Design review of the part built by this model. Coordinates are the model's own, in mm. A direction names the side the tool comes from. Round coordinates to 2 decimals unless told otherwise and drop trailing zeros. Order: outer loops, then holes, each group sorted by start corner. A loop starts at its lowest first (then second) coordinate and runs counter-clockwise, first axis right, second up.
Autodesk Inventor part; units mm, degrees
ref_plane "YZ Plane" through (0, 0, 0) normal (1, 0, 0) x (0, 1, 0)
ref_plane "XZ Plane" through (0, 0, 0) normal (0, 1, 0) x (-1, 0, 0)
ref_plane "XY Plane" through (0, 0, 0) normal (0, 0, 1) x (1, 0, 0)
sketch "Sketch4" plane through (0, 0, 0) normal (1, 0, 0) x (0, 1, 0)
  line L0 (0, 0) -> (3, 0)
  line L1 (3, 0) -> (3, -4.5)
  line L2 (3, -4.5) -> (0, -4.5)
  line L3 (0, -4.5) -> (0, 0)
  dimension "d21" = 3
  dimension "d22" = 4.5
extrude "Extrusion2" add sketch "Sketch4" along normal blind 100
sketch "Sketch5" plane through (0, 3, 0) normal (0, 1, 0) x (1, 0, 0)
  circle A0 centre (2.25, 2.25) radius 1.5
  circle A1 centre (96.8723, 2.25) radius 1.5
  line L0 (0, 4.5) -> (0, 0) construction
  line L1 (0, 0) -> (100, 0) construction
  dimension "d25" = 3
  dimension "d26" = 3
  dimension "d27" = 2.25
  dimension "d28" = 2.25
  dimension "d29" = 4.5
hole "Hole2" at (2.25, 3, -2.25) at (96.8723, 3, -2.25) direction (0, -1, 0) diameter 3.4 depth 8.8 tip angle 118
sketch "Sketch6" plane through (0, 3, 0) normal (0, 1, 0) x (1, 0, 0)
  line L0 (7.5, 1.15) -> (92.5, 1.15)
  line L1 (92.5, 1.15) -> (92.5, 3.35)
  line L2 (92.5, 3.35) -> (7.5, 3.35)
  line L3 (7.5, 3.35) -> (7.5, 1.15)
  line L4 (0, 4.5) -> (100, 4.5)
  line L5 (0, 0) -> (100, 0)
  line L6 (0, 4.5) -> (0, 0)
  dimension "d37" = 85
  dimension "d38" = 2.2
  dimension "d39" = 4.5
  dimension "d40" = 1.15
  dimension "d41" = 7.5
extrude "Extrusion3" cut sketch "Sketch6" against normal blind 100
sketch "Sketch7" plane through (0, 0, 0) normal (0, 0, 1) x (1, 0, 0)
  line L0 (0, 0) -> (100, 0)
  line L1 (100, 0) -> (100, 3)
  line L2 (100, 3) -> (0, 3)
  line L3 (0, 3) -> (0, 0)
extrude "Extrusion4" add sketch "Sketch7" along normal blind 8
sketch "Sketch8" plane through (0, 3, -4.5) normal (0, 1, 0) x (1, 0, 0)
  line L0 (11, -9.5) -> (89, -9.5) construction
  line L1 (0, 0) -> (0, -12.5)
  line L2 (-1, -16) -> (89, -16) construction
  line L3 (-1, -17) -> (89, -17) construction
  line L4 (89, -15) -> (-1, -15) construction
  arc A0 (-1, -15) -> (-1, -17) centre (-1, -16) ccw construction
  arc A1 (89, -17) -> (89, -15) centre (89, -16) ccw construction
  circle A2 centre (11, -9.5) radius 1
  circle A3 centre (89, -9.5) radius 1
  circle A4 centre (82.5, -9.5) radius 1
  circle A5 centre (17.5, -9.5) radius 1
  point P0 (0, -4.5)
  point P1 (50, -9.5)
  point P2 (44, -16)
  dimension "d47" = 78
  dimension "d48" = 50
  dimension "d49" = 2
  dimension "d50" = 90
  dimension "d51" = 6.5
  dimension "d54" = 9.5
  dimension "d55" = 2
  dimension "d56" = 2
  dimension "d57" = 2
  dimension "d58" = 2
  dimension "d59" = 6.5
  dimension "d60" = 6.5
sketch "Sketch9" plane through (0, 0, -4.5) normal (0, -1, 0) x (1, 0, 0)
  point P0 (0, 4.5)
sketch "Sketch10" plane through (0, 0, -4.5) normal (0, -1, 0) x (1, 0, 0)
  point P0 (0, 4.5)
hole "Hole3" at (11, 3, 5) at (17.5, 3, 5) at (82.5, 3, 5) at (89, 3, 5) direction (0, -1, 0) diameter 1.221 depth 5.3 tip angle 118
chamfer "Chamfer1" distance 0.1 angle 45 4 edges at (11, 3, 4.3895) (17.5, 3, 4.3895) (82.5, 3, 4.3895) (89, 3, 4.3895)
equation "\"d27\" = d28"
equation "\"d28\" = 0.5 * d29"
properties part number "szyna"
1) Take a section at C-C on y = 0.85. Give the boundary of the cut face in (x, z).
Results:
outline: (0, -4.5) - (100, -4.5) - (100, 8) - (0, 8) - close; hole circle Ø3.4 at (2.25, -2.25); hole (7.5, -3.35) - (92.5, -3.35) - (92.5, -1.15) - (7.5, -1.15) - close; hole circle Ø1.22 at (11, 5); hole circle Ø1.22 at (17.5, 5); hole circle Ø1.22 at (82.5, 5); hole circle Ø1.22 at (89, 5); hole circle Ø3.4 at (96.87, -2.25)
2) For faces 4 (the face through (49, 0, 2)), 5 (the face through (7.5, 2, -2)), list the 3-axis set-ups (+Z, -Z, +X, -X, +Y, -Y) from which the entire face can be reached by the end or side of a thin tool; tool diameter is ignored.
Results:
face 4: +Z, -Z, +X, -X, -Y
face 5: +Y, -Y
3) The part is to be moulded in two halves that separate along X. For faces 1 (the face through (0, 2, 2)), 2 (the face through (51, 2, -3.35)), 3 (the face through (49, 2, 8)), say which applies: released by +X, released by -X, zero draft, split by the parting line, or undercut.
Results:
face 1: released by -X
face 2: undercut
face 3: zero draft
4) Take a section at B-B on z = -2.25. Give the boundary of the cut face in (x, y), plus the area to 3 significant figures.
Results:
outline: (0, 0) - (0.55, 0) - (0.55, 3) - (0, 3) - close; (3.95, 0) - (7.5, 0) - (7.5, 3) - (3.95, 3) - close; (92.5, 0) - (95.17, 0) - (95.17, 3) - (92.5, 3) - close; (98.57, 0) - (100, 0) - (100, 3) - (98.57, 3) - close
area: 24.6 mm2
5) Clearance check with a flat-ended pin moving along its axis: P1, Ø4, axis at x = 50.5, z = -3, coming from the +Y side. State where the tip first meets the part, or that it passes through.
Results:
P1: stops at y = 3
6) Take a section at D-D on x = 74. Give the boundary of the cut face in (y, z).
Results:
outline: (0, -4.5) - (3, -4.5) - (3, -3.35) - (0, -3.35) - close; (0, -1.15) - (3, -1.15) - (3, 8) - (0, 8) - close
7) Take a section at A-A on x = 2.25. Give the boundary of the cut face in (y, z).
Results:
outline: (0, -4.5) - (3, -4.5) - (3, -3.95) - (0, -3.95) - close; (0, -0.55) - (3, -0.55) - (3, 8) - (0, 8) - close
8) To check wall thickness, follow line 1 along X through (y, z) = (1.9, 5); line 2 along X through (y, z) = (1.55, -2.25); line 3 along Z through (x, y) = (17.5, 1.5). State the ranges of each line that lie inside material, in increasing order.
Results:
line 1: x = 0 to 10.39, 11.61 to 16.89, 18.11 to 81.89, 83.11 to 88.39, 89.61 to 100
line 2: x = 0 to 0.55, 3.95 to 7.5, 92.5 to 95.17, 98.57 to 100
line 3: z = -4.5 to -3.35, -1.15 to 4.39, 5.61 to 8
